```python
from build123d import *

# Parameters (mm, degrees)
SKETCH1_W                    = 17.7
SKETCH1_H                    = 60
BASE_FLANGE2_DEPTH           = 2
EDGE_FLANGE2_STRIP_W         = 9.4732
EDGE_FLANGE2_STRIP_H         = 2
EDGE_FLANGE2_STRIP_CUT_DEPTH = 60
EDGE_FLANGE2_DEPTH           = 60
CUT_EXTRUDE5_DEPTH           = 2
FILLET4_R                    = 5
FILLET5_R                    = 3
SKETCH22_R                   = 2
CUT_EXTRUDE6_DEPTH           = 2
CUT_EXTRUDE7_DEPTH           = 2
FILLET6_R                    = 1


# Sheet-metal steps are written as plain solids
with BuildPart() as part:
    # Sketch1 → Base-Flange2 (new body)
    with BuildSketch(Plane(origin=(0, 0, 0), x_dir=(1, 0, 0), z_dir=(0, 1, 0))):
        with Locations((-8.85, -30)):
            Rectangle(SKETCH1_W, SKETCH1_H)
    extrude(amount=-BASE_FLANGE2_DEPTH)

    # Edge-Flange2 strip (across the edge) → Edge-Flange2 strip cut (cut)
    with BuildSketch(Plane(origin=(-17.7, -2, 60), x_dir=(1, 0, 0), z_dir=(0, 0, -1))):
        with Locations((-4, -1)):
            Rectangle(EDGE_FLANGE2_STRIP_W, EDGE_FLANGE2_STRIP_H)
    extrude(amount=EDGE_FLANGE2_STRIP_CUT_DEPTH, mode=Mode.SUBTRACT)

    # Edge-Flange2 section (across the edge) → Edge-Flange2 (add)
    with BuildSketch(Plane(origin=(-17.7, -2, 60), x_dir=(1, 0, 0), z_dir=(0, 0, -1))):
        with BuildLine():
            Line((-2, 0.7366), (-2, 20))
            Line((-2, 20), (0, 20))
            Line((0, 20), (0, 0.7366))
            ThreePointArc((0, 0.7366), (0.215745145, 0.215745145), (0.7366, 0))
            Line((0.7366, 0), (0.7366, -2))
            ThreePointArc((0.7366, -2), (-1.198468417, -1.198468417), (-2, 0.7366))
        make_face()
    extrude(amount=EDGE_FLANGE2_DEPTH)

    # Sketch20 → Cut-Extrude5 (cut)
    with BuildSketch(Plane.ZY.offset(19.7)):
        Polygon((0, -5), (40, -22), (0, -22), align=None)
    extrude(amount=-CUT_EXTRUDE5_DEPTH, mode=Mode.SUBTRACT)

    # Fillet4
    fillet4_edges = [part.edges().sort_by_distance(p)[0] for p in [
        (-18.7, -22, 60),
        (-18.7, -22, 40),
    ]]
    fillet(fillet4_edges, radius=FILLET4_R)

    # Fillet5
    fillet5_edges = [part.edges().sort_by_distance(p)[0] for p in [
        (-18.7, -5, 0),
    ]]
    fillet(fillet5_edges, radius=FILLET5_R)

    # Sketch22 → Cut-Extrude6 (cut)
    with BuildSketch(Plane.ZY.offset(19.7)):
        with Locations(Location((54, -16, 0), (0, 0, 270))):
            Circle(SKETCH22_R)
    extrude(amount=-CUT_EXTRUDE6_DEPTH, mode=Mode.SUBTRACT)

    # Mirror1: part across plane


with BuildPart() as part_1:
    add(part.part)
    add(part.part.mirror(Plane(origin=(0, -2, 60), x_dir=(0, 0, 1), z_dir=(1, 0, 0))))

    # Sketch28 → Cut-Extrude7 (cut)
    with BuildSketch(Plane(origin=(0, 0, 0), x_dir=(1, 0, 0), z_dir=(0, 1, 0))):
        with BuildLine():
            Line((2, -55), (2, -60))
            Line((2, -60), (-2, -60))
            Line((-2, -60), (-2, -55))
            ThreePointArc((-2, -55), (0, -53), (2, -55))
        make_face()
    extrude(amount=-CUT_EXTRUDE7_DEPTH, mode=Mode.SUBTRACT)

    # Fillet6
    fillet6_edges = [part_1.edges().sort_by_distance(p)[0] for p in [
        (2, -1, 60),
        (-2, -1, 60),
    ]]
    fillet(fillet6_edges, radius=FILLET6_R)


solid = part_1.part
```
Geometry check sheet. Reference: the model listing, model coordinates, mm. A direction names the side the tool comes from. Give positions to 0.01 mm unless a question says otherwise; leave off trailing zeros. Write each loop counter-clockwise with the first axis right and the second up, starting at its lowest first coordinate (ties: lowest second). Pieces come first, ordered by that corner, then holes. Notation, with made-up numbers: (14.25, 75) -> (32.25, 75) arc R20 ccw to (32.25, 110) -> close; hole circle Ø10 at (82, 41). An arc over 180 degrees is marked (long way). One line per question, with ' | ' between items.
Item 1: Sectioned sample at B-B, the plane z = 26. Record the boundary of the cut face in (x, y).
Determined:
outline: (-19.7, -16.05) -> (-17.7, -16.05) -> (-17.7, -2.74) arc R0.74 cw to (-16.96, -2) -> (16.96, -2) arc R0.74 cw to (17.7, -2.74) -> (17.7, -16.05) -> (19.7, -16.05) -> (19.7, -2.74) arc R2.74 ccw to (16.96, 0) -> (-16.96, 0) arc R2.74 ccw to (-19.7, -2.74) -> close
Item 2: Draft check along Y on faces 3 (the cylindrical face through (-19, -16, 56)), 4 (the flat face through (-18, -5, 60)), 5 (the cylindrical face through (-18.686, -4.65, 0.485)). Enter one of: released by +Y, released by -Y, zero draft, split by the parting line, or undercut.
Determined:
face 3: undercut | face 4: zero draft | face 5: released by -Y
Item 3: Access from +Z, -Z, +X, -X, +Y, -Y to the whole of each face (thin tool, end or side, straight path). Record for faces 1 (the flat face through (2, -1, 57)), 2 (the flat face through (19.7, -10, 37)).
Determined:
face 1: +Z, +Y, -Y | face 2: +Z, -Z, +X, +Y, -Y
Item 4: Sectioned sample at D-D, the plane y = -11.25. Record the boundary of the cut face in (x, z), plus the area to 3 significant figures.
Determined:
outline: (-19.7, 14.71) -> (-17.7, 14.71) -> (-17.7, 60) -> (-19.7, 60) -> close; (17.7, 14.71) -> (19.7, 14.71) -> (19.7, 60) -> (17.7, 60) -> close | area: 181 mm^2
Item 5: Sectioned sample at A-A, the plane z = 54. Record the boundary of the cut face in (x, y).
Determined:
outline: (-19.7, -22) -> (-17.7, -22) -> (-17.7, -18) -> (-19.7, -18) -> close; (-19.7, -14) -> (-17.7, -14) -> (-17.7, -2.74) arc R0.74 cw to (-16.96, -2) -> (-1.73, -2) -> (-1.73, 0) -> (-16.96, 0) arc R2.74 ccw to (-19.7, -2.74) -> close; (1.73, -2) -> (16.96, -2) arc R0.74 cw to (17.7, -2.74) -> (17.7, -14) -> (19.7, -14) -> (19.7, -2.74) arc R2.74 ccw to (16.96, 0) -> (1.73, 0) -> close; (17.7, -22) -> (19.7, -22) -> (19.7, -18) -> (17.7, -18) -> close
Item 6: Sectioned sample at C-C, the plane y = -16. Record the boundary of the cut face in (x, z), plus the area to 3 significant figures.
Determined:
outline: (-19.7, 25.88) -> (-17.7, 25.88) -> (-17.7, 52) -> (-19.7, 52) -> close; (-19.7, 56) -> (-17.7, 56) -> (-17.7, 60) -> (-19.7, 60) -> close; (17.7, 25.88) -> (19.7, 25.88) -> (19.7, 52) -> (17.7, 52) -> close; (17.7, 56) -> (19.7, 56) -> (19.7, 60) -> (17.7, 60) -> close | area: 120 mm^2
Item 7: Depth check by flat-ended pin: pin 1 (3.5 mm diameter, centred on y = -16, z = 54, fed in from +X); pin 2 (0.6 mm diameter, centred on y = -1.5, z = 57.5, fed in from -X); pin 3 (4 mm diameter, centred on x = 2, z = 46.5, fed in from -Y); pin 4 (1 mm diameter, centred on y = -0.5, z = 57, fed in from +X). Enter the tip coordinate at first touch or a pass-through.
Determined:
pin 1: through | pin 2: x = -19.53 | pin 3: y = -2 | pin 4: x = 19.08
Item 8: Scan lines: line 1 along X through (y, z) = (-7, 32); line 2 along Y through (x, z) = (-13, 37.5); line 3 along Z through (x, y) = (0, -0.75). Record each from-to range of solid material in increasing order.
Determined:
line 1: -19.7 to -17.7, 17.7 to 19.7 | line 2: -2 to 0 | line 3: 0 to 53
